Verification items for the finished model (mm, model axes). Face numbers are marked on the shaded views. A direction names the side the tool comes from. Coordinates: 2 decimals unless noted, no trailing zeros. Order: outer loops, then holes, each group sorted by start corner. A loop starts at its lowest first (then second) coordinate and runs counter-clockwise, first axis right, second up. Notation, with made-up numbers: (58.5, 26) -> (69.5, 26) arc R21 cw to (69.5, 60) -> close; hole circle Ø9 at (83, 28.5). An arc over 180 degrees is marked (long way). Write item = value, one per line. Start each with the question number.
1. Set-up check for the marked faces 1 and 2: record each of +Z, -Z, +X, -X, +Y, -Y from which the full face is reachable in a straight line by a thin tool's end or side.
2. Thickness scan on line 1 along Y through (x, z) = (2156.75, 710); line 2 along Y through (x, z) = (2161.75, 711); line 3 along X through (y, z) = (607, 716). Record the ranges inside material, lowest first. Write a range as from..to.
3. Cross-section at A-A on y = 613. Record the cut outline in (x, z), plus the area to 3 significant figures.
4. Go/stop test with flat-tipped pins: P1, Ø12, axis at x = 2164, y = 614.5, coming from the +Z side; P2, Ø12, axis at x = 2166.5, y = 603, coming from the -Z side; P3, Ø1.5, axis at x = 2156.5, y = 600.5, coming from the -Z side. Record where each tip stops, or that it passes through.
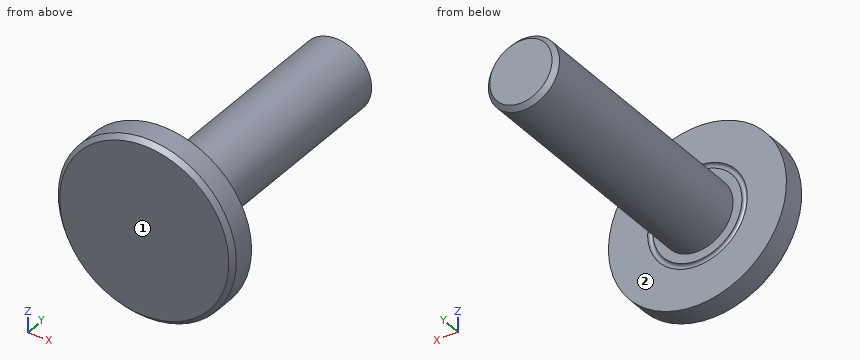
from build123d import *


with BuildPart() as part:
    # Esquisse1 → Base-Révolution (revolve)
    with BuildSketch(Plane(origin=(0, 0, 716.131939029), x_dir=(-1, 0, 0), z_dir=(0, 0, -1)), mode=Mode.PRIVATE) as base_r_volution_sk:
        with BuildLine():
            Line((-2169.949576888, 588.734614361), (-2160.449576888, 588.734614361))
            Line((-2160.449576888, 588.734614361), (-2160.449576888, 620.734614361))
            Line((-2160.449576888, 620.734614361), (-2163.949576888, 620.734614361))
            Line((-2163.949576888, 620.734614361), (-2164.449576888, 620.234614361))
            Line((-2164.449576888, 620.234614361), (-2164.449576888, 605.534359442))
            Line((-2164.449576888, 605.534359442), (-2164.449576888, 591.734359161))
            Line((-2164.449576888, 591.734359161), (-2165.449576888, 591.734359161))
            ThreePointArc((-2165.449576888, 591.734359161), (-2165.749653787, 591.434359171), (-2166.049576849, 591.734512958))
            Line((-2166.049576849, 591.734512958), (-2170.449576888, 591.734512958))
            Line((-2170.449576888, 591.734512958), (-2170.449576888, 589.234614361))
            Line((-2170.449576888, 589.234614361), (-2169.949576888, 588.734614361))
        make_face()
    revolve(base_r_volution_sk.sketch.rotate(Axis((2160.449576888, 588.734614361, 716.131939029), (0, 1, 0)), 90), axis=Axis((2160.449576888, 588.734614361, 716.131939029), (0, 1, 0)))


solid = part.part
Worked out:
q1.face_1 = +Z, -Z, +X, -X, -Y
q1.face_2 = +Y
q2.line_1 = 588.73..591.73
q2.line_2 = 588.73..591.43
q2.line_3 = 2156.45..2164.45
q3.outline = circle Ø8 at (2160.45, 716.13)
q3.area = 50.3 mm²
q4.P1 = 720.13
q4.P2 = 712.13
q4.P3 = 713.73
